from build123d import *

# Parameters (mm, degrees)
SKETCH1_W               = 71.12
SKETCH1_H               = 50.8
BOSS_EXTRUDE1_DEPTH     = 5.715
SKETCH3_R               = 3.81
SKETCH3_W               = 55.88
SKETCH3_H               = 12.7
BOSS_EXTRUDE2_DEPTH     = 3.81
F_4_40_TAPPED_HOLE1_D   = 2.2606
BOSS_EXTRUDE4_DEPTH     = 3.81
FILLET1_R               = 12.7
FILLET2_R               = 1.27
CUT_EXTRUDE1_DEPTH      = 2.54
CUT_EXTRUDE1_DEPTH_BACK = 88.917120204
SKETCH9_R               = 3.175


with BuildPart() as part:
    # Sketch1 → Boss-Extrude1 (new body)
    with BuildSketch(Plane.XY):
        with Locations((35.56, 25.4)):
            Rectangle(SKETCH1_W, SKETCH1_H)
    extrude(amount=BOSS_EXTRUDE1_DEPTH)

    # Sketch3 → Boss-Extrude2 (add)
    with BuildSketch(Plane.XY.offset(5.715)):
        with Locations(Location((19.05, 39.37, 0), (0, 0, 180))):
            Circle(SKETCH3_R)
        with Locations(Location((66.04, 39.37, 0), (0, 0, 180))):
            Circle(SKETCH3_R)
        with Locations(Location((6.35, 6.35, 0), (0, 0, 180))):
            Circle(SKETCH3_R)
        with Locations(Location((66.04, 6.35, 0), (0, 0, 180))):
            Circle(SKETCH3_R)
        with Locations((38.1, 22.86)):
            Rectangle(SKETCH3_W, SKETCH3_H)
    extrude(amount=BOSS_EXTRUDE2_DEPTH)

    # #4-40 Tapped Hole1 (through all)
    with Locations(Plane(origin=(0, 0, 0), x_dir=(-1, 0, 0), z_dir=(0, 0, -1))):
        with Locations((-66.04, 6.35), (-66.04, 39.37), (-19.05, 39.37), (-6.35, 6.35)):
            Hole(F_4_40_TAPPED_HOLE1_D / 2)

    # Sketch7 → Boss-Extrude4 (add)
    with BuildSketch(Plane.XY.offset(5.715)):
        with BuildLine():
            Line((15.24, 39.37), (15.24, 29.21))
            Line((15.24, 29.21), (22.86, 29.21))
            Line((22.86, 29.21), (22.86, 39.37))
            ThreePointArc((22.86, 39.37), (19.05, 35.56), (15.24, 39.37))
        make_face()
        with BuildLine():
            Line((62.23, 39.37), (62.23, 29.21))
            Line((62.23, 29.21), (66.04, 29.21))
            Line((66.04, 29.21), (69.571964529, 37.94125))
            ThreePointArc((69.571964529, 37.94125), (65.31222423, 35.630154759), (62.23, 39.37))
        make_face()
        with BuildLine():
            Line((3.479452055, 8.855205479), (10.16, 16.51))
            Line((10.16, 16.51), (20.273818182, 16.51))
            Line((20.273818182, 16.51), (9.220547945, 3.844794521))
            ThreePointArc((9.220547945, 3.844794521), (8.855205479, 9.220547945), (3.479452055, 8.855205479))
        make_face()
        with BuildLine():
            Line((62.23, 6.35), (62.23, 16.51))
            Line((62.23, 16.51), (66.04, 16.51))
            Line((66.04, 16.51), (69.571964529, 7.77875))
            ThreePointArc((69.571964529, 7.77875), (65.31222423, 10.089845241), (62.23, 6.35))
        make_face()
    extrude(amount=BOSS_EXTRUDE4_DEPTH)

    # Fillet1
    # the kernel refuses this fillet: 12.7 mm, written as the material it adds along each edge
    with BuildSketch(Plane(origin=(10.16, 16.51, -6.19125), x_dir=(0, 1, 0), z_dir=(0, 0, 1))) as fillet1_piece_1_section:
        with BuildLine():
            CenterArc((FILLET1_R * 0.375, FILLET1_R), FILLET1_R, 228.887909561, 41.112090439)
            Line((-FILLET1_R * 0.282534246575, FILLET1_R * 0.246575342466), (0, 0))
            Line((0, 0), (FILLET1_R * 0.375, 0))
        make_face()
    fillet1_piece_1 = extrude(amount=15.71625, mode=Mode.PRIVATE)
    fillet1_piece_1 = split(fillet1_piece_1, bisect_by=Plane(origin=(9.519597121, 16.75015108, 0), z_dir=(0, 0, 1)), keep=Keep.TOP, mode=Mode.PRIVATE)
    add(fillet1_piece_1)
    with BuildSketch(Plane(origin=(15.24, 29.21, -19.685), x_dir=(0, 1, 0), z_dir=(0, 0, 1))) as fillet1_piece_2_section:
        with BuildLine():
            CenterArc((10.16, 12.7), FILLET1_R, 216.869897646, 53.130102354)
            Line((0, 5.08), (-1.016, 4.318))
            ThreePointArc((-1.016, 4.318), (-1.27, 2.54), (-1.27, 0))
            Line((-1.27, 0), (0, -1.27))
            Line((0, -1.27), (10.16, -1.27))
            Line((10.16, -1.27), (10.16, 0))
        make_face()
    fillet1_piece_2 = extrude(amount=29.21, mode=Mode.PRIVATE)
    fillet1_piece_2 = split(fillet1_piece_2, bisect_by=Plane(origin=(13.921943776, 33.679028112, 0), z_dir=(0, 0, 1)), keep=Keep.TOP, mode=Mode.PRIVATE)
    add(fillet1_piece_2)
    with BuildSketch(Plane(origin=(62.23, 29.21, -25.543613437), x_dir=(0.0042208920727075105, 0.9999910919953791, 0), z_dir=(0, 0, 1))) as fillet1_piece_3_section:
        with BuildLine():
            CenterArc((12.647111175, 12.556939323), FILLET1_R, 180.24184002, 81.150116902)
            Line((-0.052775693, 12.503333994), (-1.32276438, 12.497973461))
            Line((-1.32276438, 12.497973461), (-1.269988687, -0.005360533))
            Line((-1.269988687, -0.005360533), (0.005360533, -1.269988687))
            ThreePointArc((0.005360533, -1.269988687), (10.165270028, -1.227104423), (10.556163414, -1.255693932))
            Line((10.556163414, -1.255693932), (10.746249574, 0))
        make_face()
    fillet1_piece_3 = extrude(amount=35.068613437, mode=Mode.PRIVATE)
    fillet1_piece_3 = split(fillet1_piece_3, bisect_by=Plane(origin=(58.003710065, 32.244364844, 0), z_dir=(0, 0, 1)), keep=Keep.TOP, mode=Mode.PRIVATE)
    add(fillet1_piece_3)
    with BuildSketch(Plane(origin=(22.86, 29.21, -25.543613437), x_dir=(1, 0, 0), z_dir=(0, 0, 1))) as fillet1_piece_4_section:
        with BuildLine():
            CenterArc((12.503445375, 12.7), FILLET1_R, 188.849883098, 81.150116902)
            Line((-0.04535876, 10.746153846), (-1.300239173, 10.550769231))
            ThreePointArc((-1.300239173, 10.550769231), (-1.27, 10.16), (-1.27, 0))
            Line((-1.27, 0), (0, -1.27))
            Line((0, -1.27), (12.503445375, -1.27))
            Line((12.503445375, -1.27), (12.503445375, 0))
        make_face()
    fillet1_piece_4 = extrude(amount=35.068613437, mode=Mode.PRIVATE)
    fillet1_piece_4 = split(fillet1_piece_4, bisect_by=Plane(origin=(27.086289935, 32.244364844, 0), z_dir=(0, 0, 1)), keep=Keep.TOP, mode=Mode.PRIVATE)
    add(fillet1_piece_4)
    with BuildSketch(Plane(origin=(62.23, 16.51, -25.543613437), x_dir=(-1, 0, 0), z_dir=(0, 0, 1))) as fillet1_piece_5_section:
        with BuildLine():
            CenterArc((12.503445375, 12.7), FILLET1_R, 188.849883098, 81.150116902)
            Line((-0.04535876, 10.746153846), (-1.300239173, 10.550769231))
            ThreePointArc((-1.300239173, 10.550769231), (-1.27, 10.16), (-1.27, 0))
            Line((-1.27, 0), (0, -1.27))
            Line((0, -1.27), (12.503445375, -1.27))
            Line((12.503445375, -1.27), (12.503445375, 0))
        make_face()
    fillet1_piece_5 = extrude(amount=35.068613437, mode=Mode.PRIVATE)
    fillet1_piece_5 = split(fillet1_piece_5, bisect_by=Plane(origin=(58.003710065, 13.475635156, 0), z_dir=(0, 0, 1)), keep=Keep.TOP, mode=Mode.PRIVATE)
    add(fillet1_piece_5)
    with BuildSketch(Plane(origin=(20.273818182, 16.51, -8.716818182), x_dir=(-0.6575342465753422, -0.7534246575342469, 0), z_dir=(0, 0, 1))) as fillet1_piece_6_section:
        with BuildLine():
            CenterArc((FILLET1_R * 0.454545454545, FILLET1_R), FILLET1_R, 221.112090439, 48.887909561)
            Line((-FILLET1_R * 0.298879202989, FILLET1_R * 0.342465753425), (0, 0))
            Line((0, 0), (FILLET1_R * 0.454545454545, 0))
        make_face()
    fillet1_piece_6 = extrude(amount=18.241818182, mode=Mode.PRIVATE)
    fillet1_piece_6 = split(fillet1_piece_6, bisect_by=Plane(origin=(20.68190581, 15.612207219, 0), z_dir=(0, 0, 1)), keep=Keep.TOP, mode=Mode.PRIVATE)
    add(fillet1_piece_6)
    with BuildSketch(Plane(origin=(66.04, 29.21, -0.463566012), x_dir=(0, -1, 0), z_dir=(0, 0, 1))) as fillet1_piece_7_section:
        with BuildLine():
            CenterArc((FILLET1_R * 0.194600504301, FILLET1_R), FILLET1_R, 247.975687163, 22.024312837)
            Line((-FILLET1_R * 0.180399495699, FILLET1_R * 0.072975189113), (0, 0))
            Line((0, 0), (FILLET1_R * 0.194600504301, 0))
        make_face()
    fillet1_piece_7 = extrude(amount=9.988566012, mode=Mode.PRIVATE)
    fillet1_piece_7 = split(fillet1_piece_7, bisect_by=Plane(origin=(66.226537553, 29.173699698, 0), z_dir=(0, 0, 1)), keep=Keep.TOP, mode=Mode.PRIVATE)
    add(fillet1_piece_7)
    with BuildSketch(Plane(origin=(66.04, 16.51, -0.463566012), x_dir=(0.37499999999999534, -0.9270248108869598, 0), z_dir=(0, 0, 1))) as fillet1_piece_8_section:
        with BuildLine():
            CenterArc((FILLET1_R * 0.194600504301, FILLET1_R), FILLET1_R, 247.975687163, 22.024312837)
            Line((-FILLET1_R * 0.180399495699, FILLET1_R * 0.072975189113), (0, 0))
            Line((0, 0), (FILLET1_R * 0.194600504301, 0))
        make_face()
    fillet1_piece_8 = extrude(amount=9.988566012, mode=Mode.PRIVATE)
    fillet1_piece_8 = split(fillet1_piece_8, bisect_by=Plane(origin=(66.226537553, 16.546300302, 0), z_dir=(0, 0, 1)), keep=Keep.TOP, mode=Mode.PRIVATE)
    add(fillet1_piece_8)

    # Fillet2
    fillet2_edges = [part.edges().sort_by_distance(p)[0] for p in [
        (10.16, 29.21, 7.62),
    ]]
    fillet(fillet2_edges, radius=FILLET2_R)

    # Sketch9 → Cut-Extrude1 (cut, two sides: drawn at the far end of the back side and taken through both)
    with BuildSketch(Plane.XY.offset(9.525).offset(-CUT_EXTRUDE1_DEPTH_BACK)):
        with Locations((25.4, 22.86)):
            Circle(SKETCH9_R)
        with Locations((50.8, 22.86)):
            Circle(SKETCH9_R)
    extrude(amount=CUT_EXTRUDE1_DEPTH + CUT_EXTRUDE1_DEPTH_BACK, mode=Mode.SUBTRACT)


solid = part.part
Verification items for the finished model (mm, model axes). A direction names the side the tool comes from. Round coordinates to 2 decimals unless told otherwise and drop trailing zeros. Loops run counter-clockwise (first coordinate to the right, second up) from the corner with the lowest first, then second, coordinate; pieces in that order, holes last. Notation, with made-up numbers: (-12.75, -29.75) - (24.25, -29.75) arc R12 cw to (24.25, -21.75) - close; hole circle Ø3 at (23.25, 62). An arc over 180 degrees is marked (long way). Use one line per item in the form item = value.
1. Section check D-D on y = 33. Record the cut outline in (x, z) (3 decimals).
A:
outline = (0, 0) - (71.12, 0) - (71.12, 5.715) - (67.573, 5.715) - (67.573, 9.525) - (58.777, 9.525) - (58.777, 5.715) - (26.313, 5.715) - (26.313, 9.525) - (13.527, 9.525) - (13.527, 5.715) - (0, 5.715) - close
2. Section check C-C on x = 50.8. Record the cut outline in (y, z) (3 decimals), and give its area (3 significant figures).
A:
outline = (0, 0) - (19.685, 0) - (19.685, 9.525) - (16.465, 9.525) - (16.465, 5.715) - (0, 5.715) - close; (26.035, 0) - (50.8, 0) - (50.8, 5.715) - (29.255, 5.715) - (29.255, 9.525) - (26.035, 9.525) - close
area = 279 mm²
3. Section check A-A on z = 3.25. Record the cut outline in (x, y) (3 decimals).
A:
outline = (0, 0) - (71.12, 0) - (71.12, 50.8) - (0, 50.8) - close; hole circle Ø2.261 at (6.35, 6.35); hole circle Ø2.261 at (19.05, 39.37); hole circle Ø6.35 at (25.4, 22.86); hole circle Ø6.35 at (50.8, 22.86); hole circle Ø2.261 at (66.04, 6.35); hole circle Ø2.261 at (66.04, 39.37)
4. Gauge pin test, flat ends, axial feed: pin 1 Ø4 at (x, y) = (50.8, 22.86) entering from +Z; pin 2 Ø2 at (y, z) = (16.5, 8) entering from +X; pin 3 Ø1.9 at (x, z) = (39.5, 7) entering from +Y; pin 4 Ø1.9 at (y, z) = (25, 7) entering from -X. Record the tip position at first contact, or that the pin passes through.
A:
pin_1 = through
pin_2 = 66.53
pin_3 = 29.21
pin_4 = 10.16
5. Section check B-B on y = 22.86. Record the cut outline in (x, z) (3 decimals), and give its area (3 significant figures).
A:
outline = (0, 0) - (22.225, 0) - (22.225, 9.525) - (10.16, 9.525) - (10.16, 5.715) - (0, 5.715) - close; (28.575, 0) - (47.625, 0) - (47.625, 9.525) - (28.575, 9.525) - close; (53.975, 0) - (71.12, 0) - (71.12, 5.715) - (66.04, 5.715) - (66.04, 9.525) - (53.975, 9.525) - close
area = 498 mm²
6. Draft check along Y on faces 1 (the flat face through (42, 29.21, 8)), 2 (the cylindrical face through (66.28, 29.2, 7.59)), 3 (the flat face through (12.9, 8.06, 7.59)). Enter one of: pulls with the +Y half, pulls with the -Y half, needs draft (parallel to the pull), parting line crosses it, or undercut.
A:
face_1 = pulls with the +Y half
face_2 = undercut
face_3 = pulls with the -Y half
7. Scan lines: probe 1 along X at (y, z) = (22.86, 3.75) (3 decimals); probe 2 along X at (y, z) = (22.86, 6.25) (3 decimals); probe 3 along X at (y, z) = (6, 8). Record each from-to range of solid material in increasing order.
A:
probe_1 = 0 to 22.225, 28.575 to 47.625, 53.975 to 71.12
probe_2 = 10.16 to 22.225, 28.575 to 47.625, 53.975 to 66.04
probe_3 = 2.56 to 5.28, 7.42 to 11.1, 62.24 to 64.97, 67.11 to 69.83
8. Access from +Z, -Z, +X, -X, +Y, -Y to the whole of each face (thin tool, end or side, straight path). Record for faces 4 (the cylindrical face through (27.008, 32.346, 7.593)), 5 (the cylindrical face through (5.517, 7.114, 4.829)), 6 (the flat face through (38, 16.51, 8)), 7 (the cylindrical face through (3.78, 3.54, 7.59)), 8 (the cylindrical face through (14, 33.9, 7.6)).
A:
face_4 = +Z, +Y
face_5 = +Z, -Z
face_6 = +Z, -Y
face_7 = +Z
face_8 = +Z, -X, +Y
